Part model, mm, in its own coordinate system. A direction names the side the tool comes from. Coordinates: 2 decimals unless noted, no trailing zeros. Loops run counter-clockwise (first coordinate to the right, second up) from the corner with the lowest first, then second, coordinate; pieces in that order, holes last. Notation, with made-up numbers: (37, 58) - (45, 58) arc R29 ccw to (45, 85) - close; hole circle Ø8 at (-1, -29). An arc over 180 degrees is marked (long way). Use a Markdown table: item, result. Add a question column.
1. Drop flat-ended pins along their axis: pin 1 (5.5 mm diameter, centred on x = 44.5, y = -4, fed in from +Z); pin 2 (1.4 mm diameter, centred on x = 19, z = 9, fed in from -Y); pin 3 (4 mm diameter, centred on x = 2.5, y = -15, fed in from -Z); pin 4 (4.5 mm diameter, centred on x = 53.54, y = -14.92, fed in from +Z). Give the stop position or say it passes through.
2. Band-saw the part on B-B, the plane y = -18.25. Give the cut face in (x, z).
3. Band-saw the part on D-D, the plane y = -5.5. Give the cut face in (x, z), plus the area to 3 significant figures.
4. Band-saw the part on A-A, the plane z = 9. Give the cut face in (x, y), plus the area to 3 significant figures.
5. 3-axis set-ups, long thin cutter, end or side, ignore diameter. For faces 4 (the flat face through (36, -5, 11.1)), 5 (the flat face through (7.576, -10, -12)), 6 (the flat face through (48, -10, -12)): which of +Z, -Z, +X, -X, +Y, -Y reach the whole face in a straight line?
6. Band-saw the part on C-C, the plane x = 47. Give the cut face in (y, z).
7. Pull direction X, two halves, no side cores. Call faces 1 (the flat face through (0, -10, 1)), 2 (the cylindrical face through (44.9, -2.2, 9.1)), 3 (the cylindrical face through (51.17, -4.84, 1.18)): pulls with the +X half, pulls with the -X half, needs draft (parallel to the pull), parting line crosses it, or undercut.
8. Wall check: probe 1 along X at (y, z) = (-6.75, -17); probe 2 along Z at (x, y) = (17.5, -2.5); probe 3 along Y at (x, z) = (31, 9). Give the ranges that are in metal, low to high. Write a range as [from, to].
from build123d import *

# Parameters (mm, degrees)
AUFSATZ_LINEAR_AUSTRAGEN1_DEPTH = 2.4
SKIZZE3_W                       = 40.5
SKIZZE3_H                       = 20
AUFSATZ_LINEAR_AUSTRAGEN2_DEPTH = 5.8
AUFSATZ_LINEAR_AUSTRAGEN3_DEPTH = 1.8
SKIZZE5_R                       = 6.5
AUFSATZ_LINEAR_AUSTRAGEN4_DEPTH = 1.1
SKIZZE7_R                       = 5.375
AUFSATZ_LINEAR_AUSTRAGEN6_DEPTH = 0.5
AUFSATZ_LINEAR_AUSTRAGEN7_DEPTH = 3.9
SKIZZE9_W                       = 40.423818814
SKIZZE9_H                       = 24.1
AUFSATZ_LINEAR_AUSTRAGEN8_DEPTH = 20


with BuildPart() as part:
    # Skizze1 → Aufsatz-Linear austragen1 (new body)
    with BuildSketch(Plane.XY):
        with BuildLine():
            Line((0, 0), (55.5, 0))
            Line((55.5, 0), (55.5, -3.573452275))
            ThreePointArc((55.5, -3.573452275), (51.16844052, -4.919743477), (55.5, -6.266034679))
            Line((55.5, -6.266034679), (55.5, -13.573452275))
            ThreePointArc((55.5, -13.573452275), (51.16844052, -14.919743477), (55.5, -16.266034679))
            Line((55.5, -16.266034679), (55.5, -20))
            Line((55.5, -20), (0, -20))
            Line((0, -20), (0, -16.266034679))
            ThreePointArc((0, -16.266034679), (4.33155948, -14.919743477), (0, -13.573452275))
            Line((0, -13.573452275), (0, -6.266034679))
            ThreePointArc((0, -6.266034679), (4.33155948, -4.919743477), (0, -3.573452275))
            Line((0, -3.573452275), (0, 0))
        make_face()
    extrude(amount=AUFSATZ_LINEAR_AUSTRAGEN1_DEPTH)

    # Skizze3 → Aufsatz-Linear austragen2 (add)
    with BuildSketch(Plane.XY.offset(2.4)):
        with Locations((27.75, -10)):
            Rectangle(SKIZZE3_W, SKIZZE3_H)
    extrude(amount=AUFSATZ_LINEAR_AUSTRAGEN2_DEPTH)

    # Skizze4 → Aufsatz-Linear austragen3 (add)
    with BuildSketch(Plane.XY.offset(8.2)):
        with BuildLine():
            Line((37.279047641, 0), (11.081933488, 0))
            Line((11.081933488, 0), (11.081933488, -19.919743477))
            Line((11.081933488, -19.919743477), (38.54344052, -19.919743477))
            ThreePointArc((38.54344052, -19.919743477), (44.352188568, -18.059672599), (48, -13.171432699))
            Line((48, -13.171432699), (48, -6.668054255))
            ThreePointArc((48, -6.668054255), (44.85616115, -2.16412885), (39.807833399, 0))
            Line((39.807833399, 0), (38.54344052, 0))
            Line((38.54344052, 0), (37.279047641, 0))
        make_face()
    extrude(amount=AUFSATZ_LINEAR_AUSTRAGEN3_DEPTH)

    # Skizze5 → Aufsatz-Linear austragen4 (add)
    with BuildSketch(Plane.XY.offset(10)):
        with Locations((38.54344052, -10)):
            Circle(SKIZZE5_R)
    extrude(amount=AUFSATZ_LINEAR_AUSTRAGEN4_DEPTH)

    # Skizze7 → Aufsatz-Linear austragen6 (add)
    with BuildSketch(Plane.XY.offset(11.1)):
        with Locations((38.54344052, -10)):
            Circle(SKIZZE7_R)
    extrude(amount=AUFSATZ_LINEAR_AUSTRAGEN6_DEPTH)

    # Skizze8 → Aufsatz-Linear austragen7 (add)
    with BuildSketch(Plane.XY.offset(11.6)):
        with BuildLine():
            ThreePointArc((41.283566191, -11.221356338), (41.332769977, -11.104373658), (41.376982116, -10.985414645))
            ThreePointArc((41.376982116, -10.985414645), (41.691335793, -10.808242133), (41.501219074, -10.501543639))
            ThreePointArc((41.501219074, -10.501543639), (41.519784624, -10.375999701), (41.533023853, -10.249782892))
            ThreePointArc((41.533023853, -10.249782892), (41.79344052, -10), (41.533023853, -9.750217108))
            ThreePointArc((41.533023853, -9.750217108), (41.519784624, -9.624000299), (41.501219074, -9.498456361))
            ThreePointArc((41.501219074, -9.498456361), (41.691335793, -9.191757867), (41.376982116, -9.014585355))
            ThreePointArc((41.376982116, -9.014585355), (41.332769977, -8.895626342), (41.283566191, -8.778643662))
            ThreePointArc((41.283566191, -8.778643662), (41.39143723, -8.434300559), (41.042898539, -8.340870828))
            ThreePointArc((41.042898539, -8.340870828), (40.970491503, -8.236644243), (40.893741134, -8.135573273))
            ThreePointArc((40.893741134, -8.135573273), (40.912588559, -7.775221906), (40.551764823, -7.771405489))
            ThreePointArc((40.551764823, -7.771405489), (40.455712489, -7.688460272), (40.356238046, -7.609651672))
            ThreePointArc((40.356238046, -7.609651672), (40.284877603, -7.255934242), (39.934440705, -7.34197094))
            ThreePointArc((39.934440705, -7.34197094), (39.820778394, -7.285518843), (39.704830223, -7.233924448))
            ThreePointArc((39.704830223, -7.233924448), (39.547745751, -6.909066322), (39.229714929, -7.079550131))
            ThreePointArc((39.229714929, -7.079550131), (39.105584463, -7.053138248), (38.980448013, -7.031999924))
            ThreePointArc((38.980448013, -7.031999924), (38.747509708, -6.756413133), (38.481868008, -7.000631929))
            ThreePointArc((38.481868008, -7.000631929), (38.355068961, -7.005919815), (38.228607015, -7.01656576))
            ThreePointArc((38.228607015, -7.01656576), (37.934451247, -6.807566435), (37.737889915, -7.110175053))
            ThreePointArc((37.737889915, -7.110175053), (37.616389537, -7.146830451), (37.496548164, -7.188591742))
            ThreePointArc((37.496548164, -7.188591742), (37.159657822, -7.059312079), (37.044527528, -7.401296507))
            ThreePointArc((37.044527528, -7.401296507), (36.935960135, -7.467016223), (36.83026941, -7.537268844))
            ThreePointArc((36.83026941, -7.537268844), (36.471812553, -7.495831961), (36.445347358, -7.855704059))
            ThreePointArc((36.445347358, -7.855704059), (36.356534637, -7.946358682), (36.271635497, -8.040688402))
            ThreePointArc((36.271635497, -8.040688402), (35.914135288, -8.08969793), (35.977998097, -8.444845611))
            ThreePointArc((35.977998097, -8.444845611), (35.91452048, -8.554738978), (35.855747449, -8.667218713))
            ThreePointArc((35.855747449, -8.667218713), (35.521666941, -8.803595204), (35.671845018, -9.131703232))
            ThreePointArc((35.671845018, -9.131703232), (35.637691036, -9.253930339), (35.608737041, -9.377492575))
            ThreePointArc((35.608737041, -9.377492575), (35.31906774, -9.592666991), (35.546124846, -9.873119133))
            ThreePointArc((35.546124846, -9.873119133), (35.54344052, -10), (35.546124846, -10.126880867))
            ThreePointArc((35.546124846, -10.126880867), (35.31906774, -10.407333009), (35.608737041, -10.622507425))
            ThreePointArc((35.608737041, -10.622507425), (35.637691036, -10.746069661), (35.671845018, -10.868296768))
            ThreePointArc((35.671845018, -10.868296768), (35.521666941, -11.196404796), (35.855747449, -11.332781287))
            ThreePointArc((35.855747449, -11.332781287), (35.91452048, -11.445261022), (35.977998097, -11.555154389))
            ThreePointArc((35.977998097, -11.555154389), (35.914135288, -11.91030207), (36.271635497, -11.959311598))
            ThreePointArc((36.271635497, -11.959311598), (36.356534637, -12.053641318), (36.445347358, -12.144295941))
            ThreePointArc((36.445347358, -12.144295941), (36.471812553, -12.504168039), (36.83026941, -12.462731156))
            ThreePointArc((36.83026941, -12.462731156), (36.935960135, -12.532983777), (37.044527528, -12.598703493))
            ThreePointArc((37.044527528, -12.598703493), (37.159657822, -12.940687921), (37.496548164, -12.811408258))
            ThreePointArc((37.496548164, -12.811408258), (37.616389537, -12.853169549), (37.737889915, -12.889824947))
            ThreePointArc((37.737889915, -12.889824947), (37.934451247, -13.192433565), (38.228607015, -12.98343424))
            ThreePointArc((38.228607015, -12.98343424), (38.355068961, -12.994080185), (38.481868008, -12.999368071))
            ThreePointArc((38.481868008, -12.999368071), (38.747509708, -13.243586867), (38.980448013, -12.968000076))
            ThreePointArc((38.980448013, -12.968000076), (39.105584463, -12.946861752), (39.229714929, -12.920449869))
            ThreePointArc((39.229714929, -12.920449869), (39.547745751, -13.090933678), (39.704830223, -12.766075552))
            ThreePointArc((39.704830223, -12.766075552), (39.820778394, -12.714481157), (39.934440705, -12.65802906))
            ThreePointArc((39.934440705, -12.65802906), (40.284877603, -12.744065758), (40.356238046, -12.390348328))
            ThreePointArc((40.356238046, -12.390348328), (40.455712489, -12.311539728), (40.551764823, -12.228594511))
            ThreePointArc((40.551764823, -12.228594511), (40.912588559, -12.224778094), (40.893741134, -11.864426727))
            ThreePointArc((40.893741134, -11.864426727), (40.970491503, -11.763355757), (41.042898539, -11.659129172))
            ThreePointArc((41.042898539, -11.659129172), (41.39143723, -11.565699441), (41.283566191, -11.221356338))
        make_face()
    extrude(amount=AUFSATZ_LINEAR_AUSTRAGEN7_DEPTH)

    # Skizze9 → Aufsatz-Linear austragen8 (add)
    with BuildSketch(Plane(origin=(0, 0, 0), x_dir=(1, 0, 0), z_dir=(0, 1, 0))):
        with Locations((27.788090593, 12.05)):
            Rectangle(SKIZZE9_W, SKIZZE9_H)
    extrude(amount=-AUFSATZ_LINEAR_AUSTRAGEN8_DEPTH)


solid = part.part
Geometry check:
| question | item | result |
|---|---|---|
| 1 | pin 1 | stops at z = 11.1 |
| 1 | pin 2 | stops at y = -19.92 |
| 1 | pin 3 | stops at z = 0 |
| 1 | pin 4 | passes through |
| 2 | outline | (0, 0) - (7.58, 0) - (7.58, -24.1) - (48, -24.1) - (48, 0) - (55.5, 0) - (55.5, 2.4) - (48, 2.4) - (48, 8.2) - (44.08, 8.2) - (44.08, 10) - (11.08, 10) - (11.08, 8.2) - (7.5, 8.2) - (7.5, 2.4) - (0, 2.4) - close |
| 3 | outline | (4.26, 0) - (7.58, 0) - (7.58, -24.1) - (48, -24.1) - (48, 0) - (51.24, 0) - (51.24, 2.4) - (48, 2.4) - (48, 8.2) - (47.51, 8.2) - (47.51, 10) - (43.23, 10) - (43.23, 11.1) - (41.48, 11.1) - (41.48, 11.6) - (35.6, 11.6) - (35.6, 11.1) - (33.85, 11.1) - (33.85, 10) - (11.08, 10) - (11.08, 8.2) - (7.5, 8.2) - (7.5, 2.4) - (4.26, 2.4) - close |
| 3 | area | 1,400 mm^2 |
| 4 | outline | (11.08, -19.92) - (38.54, -19.92) arc R10 ccw to (48, -13.17) - (48, -6.67) arc R10 ccw to (39.81, 0) - (11.08, 0) - close |
| 4 | area | 702 mm^2 |
| 5 | face 4 | +Z |
| 5 | face 5 | -Z, -X, +Y, -Y |
| 5 | face 6 | -Z, +X, +Y, -Y |
| 6 | outline | (-20, -24.1) - (0, -24.1) - (0, 8.2) - (-4.58, 8.2) - (-4.58, 10) - (-15.26, 10) - (-15.26, 8.2) - (-20, 8.2) - close |
| 7 | face 1 | pulls with the -X half |
| 7 | face 2 | pulls with the +X half |
| 7 | face 3 | undercut |
| 8 | probe 1 | x = [7.58, 48] |
| 8 | probe 2 | z = [-24.1, 10] |
| 8 | probe 3 | y = [-19.92, 0] |
